```python
from build123d import *

# Parameters (mm, degrees)
SKETCH_1_W      = 292
SKETCH_1_H      = 125.5
EXTRUDE_1_DEPTH = 1


with BuildPart() as part:
    # 스케치1 → 보스-돌출1 (new body)
    with BuildSketch(Plane.XY):
        with BuildLine():
            Line((-328.5, 162.5), (-0.5, 162.5))
            ThreePointArc((-0.5, 162.5), (-0.146446609, 162.353553391), (0, 162))
            Line((0, 162), (0, 0.5))
            ThreePointArc((0, 0.5), (-0.146446609, 0.146446609), (-0.5, 0))
            Line((-0.5, 0), (-328.5, 0))
            ThreePointArc((-328.5, 0), (-328.853553391, 0.146446609), (-329, 0.5))
            Line((-329, 0.5), (-329, 162))
            ThreePointArc((-329, 162), (-328.853553391, 162.353553391), (-328.5, 162.5))
        make_face()
        with Locations((-164.5, 81.25)):
            Rectangle(SKETCH_1_W, SKETCH_1_H, mode=Mode.SUBTRACT)
    extrude(amount=EXTRUDE_1_DEPTH)


solid = part.part
```
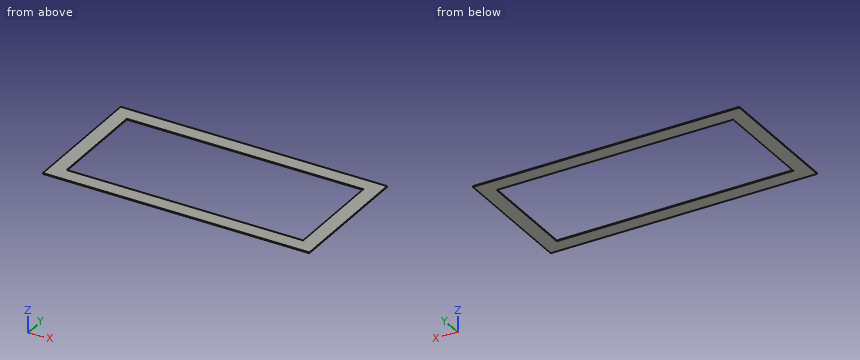
CAD build for the part. Positions are in the model's coordinates, mm. Round coordinates to 2 decimals unless told otherwise and drop trailing zeros. Write each loop counter-clockwise with the first axis right and the second up, starting at its lowest first coordinate (ties: lowest second). Pieces come first, ordered by that corner, then holes. Notation, with made-up numbers: (-17, 19.25) -> (0, 19.25) arc R16 cw to (0, 50.25) -> close; hole circle Ø2 at (55, 70.5). An arc over 180 degrees is marked (long way). Answer in a Markdown table with one row per item. Add a question column.
Item 1: Saw through at C-C, the plane z = 0.35. Write the cut outline in (x, y).
Item 2: Saw through at B-B, the plane y = 141. Write the cut outline in (x, z), then the cut area to 3 significant figures.
Item 3: Drill centre lines: line 1 (X direction, y = 85, z = 0.15); line 2 (Y direction, x = -126, z = 0.75). Where is each one in solid material? Low to high. Write a range as from..to.
Item 4: Saw through at A-A, the plane x = -222.5. Write the cut outline in (y, z).
Item 5: Drop a flat-ended pin along its axis: pin 1 Ø10 at (x, y) = (-99.5, 26) entering from -Z. Give the stop position or say it passes through.
Findings below:
| question | item | result |
|---|---|---|
| 1 | outline | (-329, 0.5) arc R0.5 ccw to (-328.5, 0) -> (-0.5, 0) arc R0.5 ccw to (0, 0.5) -> (0, 162) arc R0.5 ccw to (-0.5, 162.5) -> (-328.5, 162.5) arc R0.5 ccw to (-329, 162) -> close; hole (-310.5, 18.5) -> (-18.5, 18.5) -> (-18.5, 144) -> (-310.5, 144) -> close |
| 2 | outline | (-329, 0) -> (-310.5, 0) -> (-310.5, 1) -> (-329, 1) -> close; (-18.5, 0) -> (0, 0) -> (0, 1) -> (-18.5, 1) -> close |
| 2 | area | 37.0 mm^2 |
| 3 | line 1 | x = -329..-310.5, -18.5..0 |
| 3 | line 2 | y = 0..18.5, 144..162.5 |
| 4 | outline | (0, 0) -> (18.5, 0) -> (18.5, 1) -> (0, 1) -> close; (144, 0) -> (162.5, 0) -> (162.5, 1) -> (144, 1) -> close |
| 5 | pin 1 | passes through |
